Autodesk Inventor part; units mm, degrees
ref_plane "YZ Plane" through (0, 0, 0) normal (1, 0, 0) x (0, 1, 0)
ref_plane "XZ Plane" through (0, 0, 0) normal (0, 1, 0) x (-1, 0, 0)
ref_plane "XY Plane" through (0, 0, 0) normal (0, 0, 1) x (1, 0, 0)
sketch "Sketch1" plane through (0, 0, 0) normal (1, 0, 0) x (0, 1, 0)
  line L0 (6.35, 15.24) -> (-6.35, 15.24)
  line L1 (-6.35, 15.24) -> (-6.35, -15.24)
  line L2 (-6.35, -15.24) -> (6.35, -15.24)
  line L3 (6.35, -15.24) -> (6.35, 15.24)
  line L4 (6.35, 15.24) -> (-6.35, -15.24) construction
  line L5 (-6.35, 15.24) -> (6.35, -15.24) construction
  point P0 (0, 0)
  dimension "d0" = 12.7
  dimension "d1" = 30.48
extrude "Extrusion1" add sketch "Sketch1" along normal blind 6.35
chamfer "Chamfer1" distance 3.175 angle 45 1 edges at (6.35, 0, 15.24)
sketch "Sketch2" plane through (6.35, 0, 0) normal (1, 0, 0) x (0, 0, -1)
  point P0 (0, 0)
  point P1 (1.5638, -0.3192)
hole "Hole1" at (6.35, -0.3192, -1.5638) direction (-1, 0, 0) diameter 3 end through all
properties part number "Cover_attachment" material "Steel, Mild"
Here's how the part is built. I have some questions about the finished solid (model axes, mm). Give positions to 0.01 mm unless a question says otherwise; leave off trailing zeros. Order: outer loops, then holes, each group sorted by start corner. A loop starts at its lowest first (then second) coordinate and runs counter-clockwise, first axis right, second up. Notation, with made-up numbers: M 88.25,-20 L 134.25,-20 A22 cw 134.25,-10 Z; hole C 33.25,-4.5 d10. An arc over 180 degrees is marked long. Answer as a JSON object with one key per item and string values. Group by question number.
1) Suppose I cut it at B-B, the plane y = 0.75. Write out the boundary of the cut face in (x, z) (3 decimals), plus the area to 3 significant figures.
2) Suppose I cut it at D-D, the plane x = 2. Write out the boundary of the cut face in (y, z).
3) Please list where these lines run through material, in increasing order: L1, parallel to Y at x = 3.5, z = -0.5; L2, parallel to Z at x = 5, y = 0.75 (3 decimals); L3, parallel to Z at x = 6.25, y = 2 (3 decimals). Write a range as [from, to].
4) We'd pull the mould along Y, two halves only. Please class faces 1 (the cylindrical face through (3.131, -1.584, -2.37)), 2 (the flat face through (4.785, -0.089, 13.63)), 3 (the flat face through (3, -6.35, 0)), 4 (the flat face through (3, 6.35, 0)): pulls with the +Y half, pulls with the -Y half, needs draft (parallel to the pull), parting line crosses it, or undercut.
5) Suppose I cut it at A-A, the plane y = 2.25. Write out the boundary of the cut face in (x, z) (3 decimals), plus the area to 3 significant figures.
6) Suppose I cut it at C-C, the plane x = 4.5. Write out the boundary of the cut face in (y, z) (3 decimals).
Results found:
{
 "1": {"outline": "M 0,-15.24 L 6.35,-15.24 L 6.35,-2.616 L 0,-2.616 Z; M 0,-0.512 L 6.35,-0.512 L 6.35,12.065 L 3.175,15.24 L 0,15.24 Z", "area": "175 mm²"},
 "2": {"outline": "M -6.35,-15.24 L 6.35,-15.24 L 6.35,15.24 L -6.35,15.24 Z; hole C -0.32,-1.56 d3"},
 "3": {"L1": "[-6.35, -1.38], [0.74, 6.35]", "L2": "[-15.24, -2.616], [-0.512, 13.415]", "L3": "[-15.24, 12.165]"},
 "4": {"face 1": "undercut", "face 2": "needs draft", "face 3": "pulls with the -Y half", "face 4": "pulls with the +Y half"},
 "5": {"outline": "M 0,-15.24 L 6.35,-15.24 L 6.35,12.065 L 3.175,15.24 L 0,15.24 Z", "area": "189 mm²"},
 "6": {"outline": "M -6.35,-15.24 L 6.35,-15.24 L 6.35,13.915 L -6.35,13.915 Z; hole C -0.319,-1.564 d3"}
}
